from build123d import *

# Parameters (mm, degrees)
SKETCH1_W                = 67.5
SKETCH1_H                = 11
SKETCH2_R                = 2.5
BOSS_EXTRUDE1_DEPTH      = 15
BOSS_EXTRUDE2_DEPTH      = 2.5
BOSS_EXTRUDE2_DEPTH_BACK = 2.5
SKETCH3_R                = 2.5
BOSS_EXTRUDE3_START      = 40
SKETCH4_R                = 2.5
BOSS_EXTRUDE3_DEPTH      = 40
BOSS_EXTRUDE4_DEPTH      = 2.5
BOSS_EXTRUDE4_DEPTH_BACK = 2.5
SKETCH5_R                = 2.5


with BuildPart() as part:
    # Sketch1 → Revolve1 (revolve)
    with BuildSketch(Plane(origin=(0, 0, 0), x_dir=(0, 0, -1), z_dir=(1, 0, 0)), mode=Mode.PRIVATE) as revolve1_sk:
        with Locations((-0.842105263, 5.5)):
            Rectangle(SKETCH1_W, SKETCH1_H)
    revolve(revolve1_sk.sketch.rotate(Axis((0, 0, 34.592105263), (0, 0, -1)), 90), axis=Axis((0, 0, 34.592105263), (0, 0, -1)))

    # Sketch2 → Boss-Extrude1 (add)
    with BuildSketch(Plane.XY.offset(34.592105263)):
        Circle(SKETCH2_R)
    extrude(amount=BOSS_EXTRUDE1_DEPTH)

    # Sketch3 → Boss-Extrude2 (add, two sides: drawn at the far end of the back side and taken through both)
    with BuildSketch(Plane(origin=(0, 0, 0), x_dir=(0, 0, -1), z_dir=(1, 0, 0)).offset(-BOSS_EXTRUDE2_DEPTH_BACK)):
        with BuildLine():
            Line((-49.592105263, 2.5), (-53.958295642, 6.364761516))
            ThreePointArc((-53.958295642, 6.364761516), (-68.092105263, 0), (-53.958295642, -6.364761516))
            Line((-53.958295642, -6.364761516), (-49.592105263, -2.5))
            Line((-49.592105263, -2.5), (-49.592105263, 2.5))
        make_face()
        with Locations((-59.592105263, 0)):
            Circle(SKETCH3_R, mode=Mode.SUBTRACT)
    extrude(amount=BOSS_EXTRUDE2_DEPTH + BOSS_EXTRUDE2_DEPTH_BACK)

    # Sketch4 → Boss-Extrude3 (add)
    with BuildSketch(Plane(origin=(0, 0, -32.907894737), x_dir=(-1, 0, 0), z_dir=(0, 0, -1)).offset(BOSS_EXTRUDE3_START)):
        with Locations(Location((0, 0, 0), (0, 0, 180))):
            Circle(SKETCH4_R)
    extrude(amount=-BOSS_EXTRUDE3_DEPTH)

    # Sketch5 → Boss-Extrude4 (add, two sides: drawn at the far end of the back side and taken through both)
    with BuildSketch(Plane(origin=(0, 0, 0), x_dir=(0, 0, -1), z_dir=(1, 0, 0)).offset(-BOSS_EXTRUDE4_DEPTH_BACK)):
        with BuildLine():
            Line((72.907894737, 2.5), (85.002754977, 7.788133487))
            ThreePointArc((85.002754977, 7.788133487), (96.907894737, 0), (85.002754977, -7.788133487))
            Line((85.002754977, -7.788133487), (72.907894737, -2.5))
            Line((72.907894737, -2.5), (72.907894737, 2.5))
        make_face()
        with Locations((88.407894737, 0)):
            Circle(SKETCH5_R, mode=Mode.SUBTRACT)
    extrude(amount=BOSS_EXTRUDE4_DEPTH + BOSS_EXTRUDE4_DEPTH_BACK)


solid = part.part
The model under review builds one solid part; all positions refer to its coordinate system, in mm. A direction names the side the tool comes from. Round coordinates to 2 decimals unless told otherwise and drop trailing zeros. Loops run counter-clockwise (first coordinate to the right, second up) from the corner with the lowest first, then second, coordinate; pieces in that order, holes last. Notation, with made-up numbers: (31.25, -35) - (78.25, -35) arc R25 cw to (78.25, -12) - close; hole circle Ø10 at (63, 88.25). An arc over 180 degrees is marked (long way). Use CSV: the item, a comma, the result in double quotes.
(1) Take a section at B-B, the plane x = -8.75. Give the boundary of the cut face in (y, z).
Working result:
outline,"(-6.67, -32.91) - (6.67, -32.91) - (6.67, 34.59) - (-6.67, 34.59) - close"
(2) Take a section at D-D, the plane x = 5.75. Give the boundary of the cut face in (y, z).
Working result:
outline,"(-9.38, -32.91) - (9.38, -32.91) - (9.38, 34.59) - (-9.38, 34.59) - close"
(3) Take a section at A-A, the plane z = 4.5. Give the boundary of the cut face in (x, y).
Working result:
outline,"circle Ø22 at (0, 0)"
(4) Take a section at C-C, the plane z = -37. Give the boundary of the cut face in (x, y).
Working result:
outline,"circle Ø5 at (0, 0)"
(5) Machinability: for faces 4 (the cylindrical face through (-2.5, -0.1, -53.2)), 5 (the flat face through (-2.5, 0.1, 56.9)), 6 (the flat face through (-0.035, 4.405, 51.745)), which of the approach directions +Z, -Z, +X, -X, +Y, -Y give a long, thin tool a straight path to every point of the face, cutting with its end or side? Answer none if there is none.
Working result:
face 4,"none"
face 5,"+Z, -X, +Y, -Y"
face 6,"+X, -X, +Y"
(6) For line 1 (Z direction, x = -0.25, y = -0.25); line 2 (Z direction, x = -1.5, y = -4.25); line 3 (Y direction, x = -7, z = 30), list the stretches that pass through material, from the lowest coordinate up.
Working result:
line 1,"z = -96.9 to -90.9, -85.92 to 57.1, 62.08 to 68.09"
line 2,"z = -95.77 to -76.91, -32.91 to 34.59, 51.57 to 66.95"
line 3,"y = -8.49 to 8.49"
(7) Clearance check with flat-ended pins moving along their axes: P1, Ø5, axis at x = -0.5, y = -5, coming from the +Z side; P2, Ø1, axis at x = -3.5, y = 6.5, coming from the +Z side; P3, Ø3, axis at x = -6, y = -3, coming from the -Z side. State where each tip first meets the part, or that it passes through.
Working result:
P1,"stops at z = 67.72"
P2,"stops at z = 34.59"
P3,"stops at z = -32.91"
(8) The part is to be moulded in two halves that separate along Y. For faces 1 (the flat face through (2.5, 0.1, 56.9)), 2 (the cylindrical face through (-0.04, 0.11, -85.91)), 3 (the flat face through (-0.035, 5.107, -78.871)), say which applies: pulls with the +Y half, pulls with the -Y half, needs draft (parallel to the pull), parting line crosses it, or undercut.
Working result:
face 1,"needs draft"
face 2,"undercut"
face 3,"pulls with the +Y half"
